Geometry: see drawing. Coordinates: mm, zero at the bounding-box minimum. A direction names the side the tool comes from. Give positions to 0.01 mm unless a question says otherwise; leave off trailing zeros. Loops run counter-clockwise (first coordinate to the right, second up) from the corner with the lowest first, then second, coordinate; pieces in that order, holes last. Notation, with made-up numbers: M 44,27.5 L 72,27.5 A26 cw 72,53.5 Z; hole C -40,-20 d6. An arc over 180 degrees is marked long. Use a Markdown table: item, result. Add a question column.
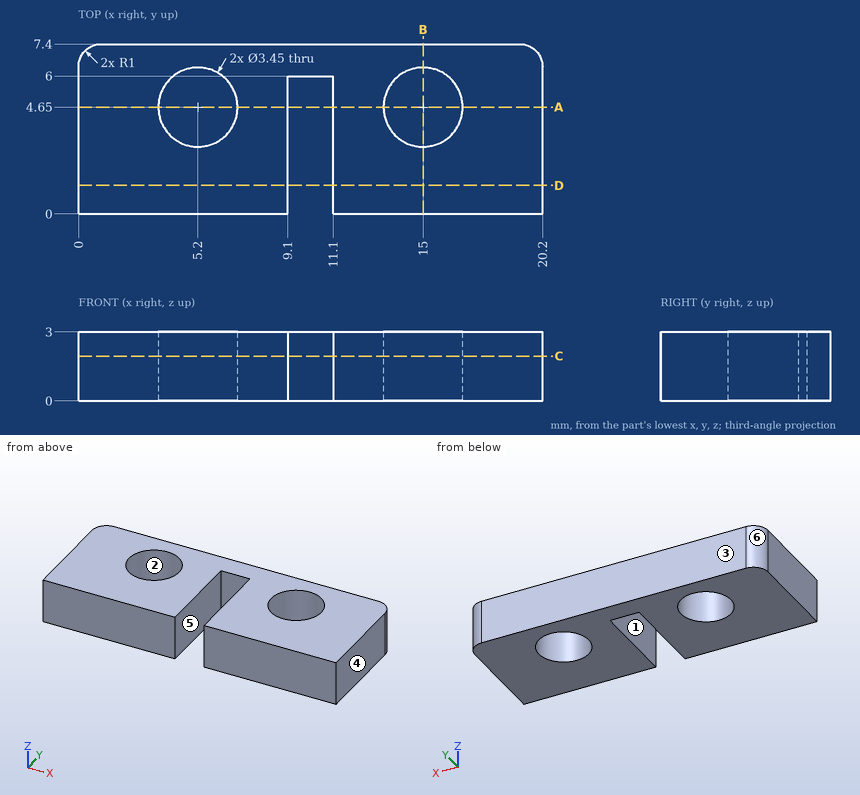
1) Section query C-C, the plane z = 1.95. Return the cut outline in (x, y) (3 decimals), and give its area (3 significant figures).
2) Section query D-D, the plane y = 1.25. Return the cut outline in (x, z), and give its area (3 significant figures).
3) Section query B-B, the plane x = 15. Return the cut outline in (y, z) (3 decimals).
4) Pull-direction query (X, two-part tool) for the marked faces 1, 2, 3 and 4; classes: pulls with the +X half, pulls with the -X half, needs draft (parallel to the pull), parting line crosses it, or undercut.
5) Ray query, line 1 (Y direction, x = 5.2, z = 1.25) (3 decimals); line 2 (X direction, y = 2, z = 2.1); line 3 (X direction, y = 4.75, z = 2.4). Return the intervals inside material, ascending. Write a range as [from, to].
6) Section query A-A, the plane y = 4.65. Return the cut outline in (x, z) (3 decimals), and give its area (3 significant figures).
7) Reachability of the marked faces 5 and 6 from +Z, -Z, +X, -X, +Y, -Y: full face, straight path, thin tool, end or side. Return the list, or none.
Entries:
| question | item | result |
|---|---|---|
| 1 | outline | M 0,0 L 9.1,0 L 9.1,6 L 11.1,6 L 11.1,0 L 20.2,0 L 20.2,6.4 A1 ccw 19.2,7.4 L 1,7.4 A1 ccw 0,6.4 Z; hole C 5.2,4.65 d3.45; hole C 15,4.65 d3.45 |
| 1 | area | 118 mm² |
| 2 | outline | M 0,0 L 9.1,0 L 9.1,3 L 0,3 Z; M 11.1,0 L 20.2,0 L 20.2,3 L 11.1,3 Z |
| 2 | area | 54.6 mm² |
| 3 | outline | M 0,0 L 2.925,0 L 2.925,3 L 0,3 Z; M 6.375,0 L 7.4,0 L 7.4,3 L 6.375,3 Z |
| 4 | face 1 | undercut |
| 4 | face 2 | undercut |
| 4 | face 3 | needs draft |
| 4 | face 4 | pulls with the +X half |
| 5 | line 1 | y = [0, 2.925], [6.375, 7.4] |
| 5 | line 2 | x = [0, 9.1], [11.1, 20.2] |
| 5 | line 3 | x = [0, 3.48], [6.92, 9.1], [11.1, 13.28], [16.72, 20.2] |
| 6 | outline | M 0,0 L 3.475,0 L 3.475,3 L 0,3 Z; M 6.925,0 L 9.1,0 L 9.1,3 L 6.925,3 Z; M 11.1,0 L 13.275,0 L 13.275,3 L 11.1,3 Z; M 16.725,0 L 20.2,0 L 20.2,3 L 16.725,3 Z |
| 6 | area | 33.9 mm² |
| 7 | face 5 | +Z, -Z, -Y |
| 7 | face 6 | +Z, -Z, -X, +Y |
